Build history of the part. All positions in model axes, mm. Face numbers are marked on the shaded views. A direction names the side the tool comes from. Give positions to 0.01 mm unless a question says otherwise; leave off trailing zeros. Loops run counter-clockwise (first coordinate to the right, second up) from the corner with the lowest first, then second, coordinate; pieces in that order, holes last. Notation, with made-up numbers: M 34.5,-38 L 84.5,-38 A20 ccw 84.5,-17 Z; hole C 81.25,-30.75 d8. An arc over 180 degrees is marked long. Answer as a JSON object with one key per item and string values. Group by question number.
1. Drill centre lines: line 1 along X through (y, z) = (-0.7, 0); line 2 along X through (y, z) = (2.1, 0); line 3 along X through (y, z) = (1.7, 14). Where is each one in solid material? Low to high. Write a range as [from, to].
2. Slice it at D-D (z = 13). List the corners of the cut face in (x, y).
3. 3-axis set-ups, long thin cutter, end or side, ignore diameter. For the marked faces 1, 2 and 3: which of +Z, -Z, +X, -X, +Y, -Y reach the whole face in a straight line?
4. Slice it at B-B (y = 0.6). List the corners of the cut face in (x, z).
5. Slice it at C-C (x = -17). List the corners of the cut face in (y, z).
6. Drop flat-ended pins along their axis: pin 1 Ø1.8 at (x, z) = (-15.5, 0) entering from +Y; pin 2 Ø2 at (x, z) = (-25, 0) entering from -Y; pin 3 Ø3 at (y, z) = (-2.5, 3.5) entering from -X; pin 4 Ø4 at (x, z) = (0, 0) entering from +Y. Give the stop position or say it passes through.
7. Slice it at A-A (z = 0). List the corners of the cut face in (x, y), then the cut area to 3 significant figures.
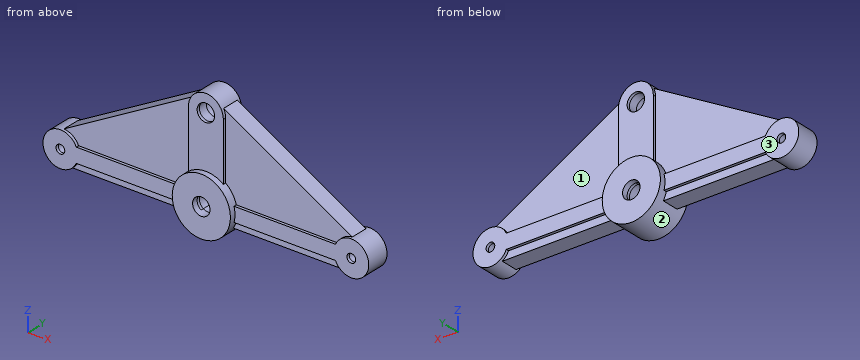
from build123d import *
from build123d.topology import SkipClean

# Parameters (mm, degrees)
SKETCH1_R      = 0.75
SKETCH1_R_2    = 1.5
EXTRUDE1_DEPTH = 1.5
SKETCH2_R      = 0.75
SKETCH2_R_2    = 1.5
EXTRUDE2_DEPTH = 2
SKETCH3_R      = 5
SKETCH3_R_2    = 1.5
EXTRUDE3_DEPTH = 3


with BuildPart() as part:
    # Sketch1 → Extrude1 (new body, symmetric)
    with BuildSketch(Plane(origin=(0, 0, 0), x_dir=(1, 0, 0), z_dir=(0, 1, 0))):
        with BuildLine():
            Line((-25, 2.5), (25, 2.5))
            ThreePointArc((25, 2.5), (27.419004196, 0.631204167), (26.221508422, -2.18126504))
            Line((26.221508422, -2.18126504), (1.221508422, -16.18126504))
            ThreePointArc((1.221508422, -16.18126504), (0, -16.5), (-1.221508422, -16.18126504))
            Line((-1.221508422, -16.18126504), (-26.221508422, -2.18126504))
            ThreePointArc((-26.221508422, -2.18126504), (-27.419004196, 0.631204167), (-25, 2.5))
        make_face()
        with Locations(Location((25, 0, 0), (0, 0, 270))):  # turned: the seam where the file's is
            Circle(SKETCH1_R, mode=Mode.SUBTRACT)
        with Locations(Location((-25, 0, 0), (0, 0, 270))):  # turned: the seam where the file's is
            Circle(SKETCH1_R, mode=Mode.SUBTRACT)
        with Locations(Location((0, -14, 0), (0, 0, 270))):  # turned: the seam where the file's is
            Circle(SKETCH1_R_2, mode=Mode.SUBTRACT)
        with Locations(Location((0, 0, 0), (0, 0, 270))):  # turned: the seam where the file's is
            Circle(SKETCH1_R_2, mode=Mode.SUBTRACT)
    extrude(amount=EXTRUDE1_DEPTH, both=True)

    # Sketch2 → Extrude2 (add, symmetric)
    with SkipClean():  # keep this step's faces unmerged: merging them makes the solid invalid here
        with BuildSketch(Plane(origin=(0, 0, 0), x_dir=(1, 0, 0), z_dir=(0, 1, 0))):
            with BuildLine():
                Line((-22.272821971, 1.25), (-0.829156198, 1.25))
                ThreePointArc((-0.829156198, 1.25), (0, -1.5), (0.829156198, 1.25))
                Line((0.829156198, 1.25), (22.272821971, 1.25))
                ThreePointArc((22.272821971, 1.25), (28, 0), (22.272821971, -1.25))
                Line((22.272821971, -1.25), (3, -1.25))
                Line((3, -1.25), (3, -14))
                ThreePointArc((3, -14), (0, -17), (-3, -14))
                Line((-3, -14), (-3, -1.25))
                Line((-3, -1.25), (-22.272821971, -1.25))
                ThreePointArc((-22.272821971, -1.25), (-28, 0), (-22.272821971, 1.25))
            make_face()
            with Locations(Location((25, 0, 0), (0, 0, 270))):  # turned: the seam where the file's is
                Circle(SKETCH2_R, mode=Mode.SUBTRACT)
            with Locations(Location((0, -14, 0), (0, 0, 270))):  # turned: the seam where the file's is
                Circle(SKETCH2_R_2, mode=Mode.SUBTRACT)
            with Locations(Location((-25, 0, 0), (0, 0, 270))):  # turned: the seam where the file's is
                Circle(SKETCH2_R, mode=Mode.SUBTRACT)
        extrude(amount=EXTRUDE2_DEPTH, both=True)

    # Sketch3 → Extrude3 (add, symmetric)
    with SkipClean():  # keep this step's faces unmerged: merging them makes the solid invalid here
        with BuildSketch(Plane(origin=(0, 0, 0), x_dir=(1, 0, 0), z_dir=(0, 1, 0))):
            with Locations(Location((0, 0, 0), (0, 0, 270))):  # turned: the seam where the file's is
                Circle(SKETCH3_R)
            with Locations(Location((0, 0, 0), (0, 0, 270))):  # turned: the seam where the file's is
                Circle(SKETCH3_R_2, mode=Mode.SUBTRACT)
        extrude(amount=EXTRUDE3_DEPTH, both=True)


solid = part.part
Established:
{
 "1": {"line 1": "x = [-28, -25.75], [-24.25, -1.5], [1.5, 24.25], [25.75, 28]", "line 2": "x = [-5, -1.5], [1.5, 5]", "line 3": "x = [-3, -1.5], [1.5, 3]"},
 "2": {"outline": "M -6.9,-1.5 L -3,-1.5 L -3,-2 L -1.12,-2 L -1.12,2 L -3,2 L -3,1.5 L -6.9,1.5 Z; M 1.12,-2 L 3,-2 L 3,-1.5 L 6.9,-1.5 L 6.9,1.5 L 3,1.5 L 3,2 L 1.12,2 Z"},
 "3": {"face 1": "+Z, +Y", "face 2": "none", "face 3": "+Z, -Z, -X, +Y"},
 "4": {"outline": "M -24.77,2.99 A3 ccw long -23.34,-2.5 L -4.33,-2.5 A5 ccw 4.33,-2.5 L 23.34,-2.5 A3 ccw long 24.77,2.99 L 2.67,15.37 A3 ccw -2.67,15.37 Z; hole C -25,0 d1.5; hole C 0,0 d3; hole C 0,14 d3; hole C 25,0 d1.5"},
 "5": {"outline": "M -2,-1.25 L -1.5,-1.25 L -1.5,-2.5 L 1.5,-2.5 L 1.5,-1.25 L 2,-1.25 L 2,1.25 L 1.5,1.25 L 1.5,7.35 L -1.5,7.35 L -1.5,1.25 L -2,1.25 Z"},
 "6": {"pin 1": "stops at y = 2", "pin 2": "stops at y = -2", "pin 3": "stops at x = -27.16", "pin 4": "stops at y = 3"},
 "7": {"outline": "M -28,-2 L -25.75,-2 L -25.75,2 L -28,2 Z; M -24.25,-2 L -5,-2 L -5,-3 L -1.5,-3 L -1.5,3 L -5,3 L -5,2 L -24.25,2 Z; M 1.5,-3 L 5,-3 L 5,-2 L 24.25,-2 L 24.25,2 L 5,2 L 5,3 L 1.5,3 Z; M 25.75,-2 L 28,-2 L 28,2 L 25.75,2 Z", "area": "214 mm^2"}
}
